Build history of the part. All positions in model axes, mm. A direction names the side the tool comes from. Round coordinates to 2 decimals unless told otherwise and drop trailing zeros. Order: outer loops, then holes, each group sorted by start corner. A loop starts at its lowest first (then second) coordinate and runs counter-clockwise, first axis right, second up. Notation, with made-up numbers: (66.5, 82.5) -> (99.5, 82.5) arc R14 ccw to (99.5, 98.5) -> close; hole circle Ø3 at (8, -5). An arc over 180 degrees is marked (long way). Use a Markdown table: item, result. Add a question column.
Item 1: Two-plate mould, pull along Y, no slides. Class faces 5 (the face through (-33, 0, -18)), 6 (the face through (-5, 1, -7)), 7 (the face through (-0.75, 0.03, -4.93)): released by +Y, released by -Y, zero draft, split by the parting line, or undercut.
Item 2: Probe L1, parallel to Y at x = -30, z = -21; L2, parallel to X at y = 0, z = -5.25. List the from-to ranges inside material, lowest first.
Item 3: Slice it at C-C, the plane x = -30. Give the cut face in (y, z), plus the area to 3 significant figures.
Item 4: Slice it at A-A, the plane z = -17.5. Give the cut face in (x, y), plus the area to 3 significant figures.
Item 5: Pin check, flat tips, straight feed: pin 1 (2.5 mm diameter, centred on x = 0, y = 0, fed in from -Z); pin 2 (7 mm diameter, centred on x = -24, z = -18.5, fed in from -Y); pin 3 (7 mm diameter, centred on x = -24, z = -18, fed in from +Y); pin 4 (1 mm diameter, centred on y = 0.5, z = -10.5, fed in from -X). Stop position of each tip, or through.
Item 6: 3-axis set-ups, long thin cutter, end or side, ignore diameter. For faces 1 (the face through (0, 0, -10)), 2 (the face through (-5, -1, -7)), 3 (the face through (-15.3, 1.8, -9.6)), 4 (the face through (-25, -1, -17)): which of +Z, -Z, +X, -X, +Y, -Y reach the whole face in a straight line?
Item 7: Slice it at B-B, the plane y = 0. Give the cut face in (x, z).
Item 8: Slice it at D-D, the plane z = -12. Give the cut face in (x, y).
from build123d import *

# Parameters (mm, degrees)
SKETCH1_R           = 3
BOSS_EXTRUDE1_DEPTH = 1
SKETCH5_R           = 0.75
CUT_EXTRUDE1_DEPTH  = 10
SKETCH6_R           = 0.75
CUT_EXTRUDE2_DEPTH  = 10


with BuildPart() as part:
    # Sweep1: sweep along a path in Sketch3
    with BuildLine(Plane(origin=(0, 0, 0), x_dir=(1, 0, 0), z_dir=(0, 1, 0))) as sweep1_path:
        Line((0, 0), (0, 12))
        Line((0, 12), (-30, 12))
        Line((-30, 12), (-30, 24))
    # Sketch1 → Sweep1 (sweep)
    with BuildSketch(Plane.XY):
        Circle(SKETCH1_R)
    sweep(path=sweep1_path.line, transition=Transition.RIGHT)

    # Sketch4 → Boss-Extrude1 (add, symmetric)
    with BuildSketch(Plane(origin=(0, 0, 0), x_dir=(1, 0, 0), z_dir=(0, 1, 0))):
        Polygon((-30, 12), (-18, 12), (-30, 24), align=None)
        Polygon((-12, 12), (0, 0), (0, 12), align=None)
    extrude(amount=BOSS_EXTRUDE1_DEPTH, both=True)

    # Sketch5 → Cut-Extrude1 (cut)
    with BuildSketch(Plane.XY):
        Circle(SKETCH5_R)
    extrude(amount=-CUT_EXTRUDE1_DEPTH, mode=Mode.SUBTRACT)

    # Sketch6 → Cut-Extrude2 (cut)
    with BuildSketch(Plane(origin=(0, 0, -24), x_dir=(-1, 0, 0), z_dir=(0, 0, -1))):
        with Locations((30, 0)):
            Circle(SKETCH6_R)
    extrude(amount=-CUT_EXTRUDE2_DEPTH, mode=Mode.SUBTRACT)


solid = part.part
Check sheet entries:
| question | item | result |
|---|---|---|
| 1 | face 5 | split by the parting line |
| 1 | face 6 | released by +Y |
| 1 | face 7 | undercut |
| 2 | L1 | -3 to -0.75, 0.75 to 3 |
| 2 | L2 | -5.25 to -0.75, 0.75 to 3 |
| 3 | outline | (-3, -24) -> (-0.75, -24) -> (-0.75, -14) -> (0.75, -14) -> (0.75, -24) -> (3, -24) -> (3, -12) arc R3 ccw to (-3, -12) -> close |
| 3 | area | 71.1 mm2 |
| 4 | outline | (-27.17, -1) -> (-23.5, -1) -> (-23.5, 1) -> (-27.17, 1) arc R3 ccw (long way) to start; hole circle Ø1.5 at (-30, 0) |
| 4 | area | 33.6 mm2 |
| 5 | pin 1 | z = -15 |
| 5 | pin 2 | y = -1.66 |
| 5 | pin 3 | y = 1.66 |
| 5 | pin 4 | x = -33 |
| 6 | face 1 | +Z |
| 6 | face 2 | +Z, -X, -Y |
| 6 | face 3 | none |
| 6 | face 4 | -Z, +X, -Y |
| 7 | outline | (-33, -24) -> (-30.75, -24) -> (-30.75, -14) -> (-29.25, -14) -> (-29.25, -24) -> (-27, -24) -> (-27, -21) -> (-21, -15) -> (3, -15) -> (3, 0) -> (0.75, 0) -> (0.75, -10) -> (-0.75, -10) -> (-0.75, 0) -> (-3, 0) -> (-3, -3) -> (-9, -9) -> (-33, -9) -> close |
| 8 | outline | (-30, -3) -> (0, -3) arc R3 ccw to (0, 3) -> (-30, 3) arc R3 ccw to start |
